Build history of the part. All positions in model axes, mm. Give positions to 0.01 mm unless a question says otherwise; leave off trailing zeros. Order: outer loops, then holes, each group sorted by start corner. A loop starts at its lowest first (then second) coordinate and runs counter-clockwise, first axis right, second up. Notation, with made-up numbers: (51.5, -10) - (98.5, -10) arc R25 cw to (98.5, 13) - close; hole circle Ø5 at (72.25, 52). An arc over 180 degrees is marked (long way). Use a Markdown table: item, result. Add a question column.
(1) Slice it at A-A (y = -449.5). Write the cut outline in (x, z), then the cut area to 3 significant figures.
(2) Slice it at C-C (z = 0.85). Count the separate pieces of the cut face and the enclosed holes in it, then the cut area to 3 significant figures.
(3) Wall check: line 1 (Y direction, x = 454, z = 1.8); line 2 (X direction, y = -454, z = 0.2); line 3 (Y direction, x = 534, z = 1.7). Give the ranges that are in metal, low to high.
(4) Mould opens along Y. For faces 1 (the face through (431, -460, 0)), 2 (the face through (323.605, -459.868, 1.479)) say: +Y half, -Y half, draft (parallel to the pull), parting line (faces both ways), or undercut.
(5) Flat gauge pin, fed straight in: pin 1 (3.5 mm diameter, centred on x = 458.79, y = -436, fed in from -Z). Where does the tip first touch, or does it go through?
(6) Slice it at B-B (x = 480). Write the cut outline in (y, z), then the cut area to 3 significant figures.
from build123d import *

# Parameters (mm, degrees)
SKETCH1_W           = 248
SKETCH1_H           = 78
SKETCH1_R           = 3.05
SKETCH1_W_2         = 24.2
SKETCH1_H_2         = 3.2
SKETCH1_W_3         = 3.2
SKETCH1_H_3         = 20.3
BOSS_EXTRUDE2_DEPTH = 3
SKETCH5_R           = 2.55
CUT_EXTRUDE1_DEPTH  = 10


with BuildPart() as part:
    # Sketch1 → Boss-Extrude2 (new body)
    with BuildSketch(Plane(origin=(0, 0, 0), x_dir=(-1, 0, 0), z_dir=(0, 0, 1))):
        with Locations((-428.787224347, 459)):
            Rectangle(SKETCH1_W, SKETCH1_H)
        with Locations(Location((-338.787224347, 436, 0), (0, 0, 180))):
            Circle(SKETCH1_R, mode=Mode.SUBTRACT)
        with Locations(Location((-368.787224347, 436, 0), (0, 0, 180))):
            Circle(SKETCH1_R, mode=Mode.SUBTRACT)
        with Locations(Location((-428.787224347, 436, 0), (0, 0, 180))):
            Circle(SKETCH1_R, mode=Mode.SUBTRACT)
        with Locations(Location((-398.787224347, 436, 0), (0, 0, 180))):
            Circle(SKETCH1_R, mode=Mode.SUBTRACT)
        with Locations(Location((-488.787224347, 436, 0), (0, 0, 180))):
            Circle(SKETCH1_R, mode=Mode.SUBTRACT)
        with Locations(Location((-458.787224347, 436, 0), (0, 0, 180))):
            Circle(SKETCH1_R, mode=Mode.SUBTRACT)
        with Locations(Location((-458.787224347, 482, 0), (0, 0, 180))):
            Circle(SKETCH1_R, mode=Mode.SUBTRACT)
        with Locations(Location((-428.787224347, 482, 0), (0, 0, 180))):
            Circle(SKETCH1_R, mode=Mode.SUBTRACT)
        with Locations(Location((-398.787224347, 482, 0), (0, 0, 180))):
            Circle(SKETCH1_R, mode=Mode.SUBTRACT)
        with Locations(Location((-368.787224347, 482, 0), (0, 0, 180))):
            Circle(SKETCH1_R, mode=Mode.SUBTRACT)
        with Locations(Location((-338.787224347, 482, 0), (0, 0, 180))):
            Circle(SKETCH1_R, mode=Mode.SUBTRACT)
        with Locations(Location((-320.787224347, 458.7, 0), (0, 0, 180))):
            Circle(SKETCH1_R, mode=Mode.SUBTRACT)
        with Locations(Location((-488.787224347, 482, 0), (0, 0, 180))):
            Circle(SKETCH1_R, mode=Mode.SUBTRACT)
        with Locations(Location((-518.787224347, 436, 0), (0, 0, 180))):
            Circle(SKETCH1_R, mode=Mode.SUBTRACT)
        with Locations(Location((-536.787224347, 459, 0), (0, 0, 180))):
            Circle(SKETCH1_R, mode=Mode.SUBTRACT)
        with Locations(Location((-518.787224347, 482, 0), (0, 0, 180))):
            Circle(SKETCH1_R, mode=Mode.SUBTRACT)
        with Locations((-383.787224347, 491.4)):
            Rectangle(SKETCH1_W_2, SKETCH1_H_2, mode=Mode.SUBTRACT)
        with Locations((-413.787224347, 491.4)):
            Rectangle(SKETCH1_W_2, SKETCH1_H_2, mode=Mode.SUBTRACT)
        with Locations((-353.787224347, 491.4)):
            Rectangle(SKETCH1_W_2, SKETCH1_H_2, mode=Mode.SUBTRACT)
        with Locations((-443.787224347, 491.4)):
            Rectangle(SKETCH1_W_2, SKETCH1_H_2, mode=Mode.SUBTRACT)
        with Locations((-473.787224347, 491.4)):
            Rectangle(SKETCH1_W_2, SKETCH1_H_2, mode=Mode.SUBTRACT)
        with Locations((-503.787224347, 491.4)):
            Rectangle(SKETCH1_W_2, SKETCH1_H_2, mode=Mode.SUBTRACT)
        with Locations((-533.787224347, 491.4)):
            Rectangle(SKETCH1_W_2, SKETCH1_H_2, mode=Mode.SUBTRACT)
        with Locations((-323.787224347, 491.4)):
            Rectangle(SKETCH1_W_2, SKETCH1_H_2, mode=Mode.SUBTRACT)
        with Locations((-313.387224347, 445.55)):
            Rectangle(SKETCH1_W_3, SKETCH1_H_3, mode=Mode.SUBTRACT)
        with Locations((-313.387224347, 471.85)):
            Rectangle(SKETCH1_W_3, SKETCH1_H_3, mode=Mode.SUBTRACT)
        with Locations((-544.187224347, 445.55)):
            Rectangle(SKETCH1_W_3, SKETCH1_H_3, mode=Mode.SUBTRACT)
        with Locations((-544.187224347, 471.85)):
            Rectangle(SKETCH1_W_3, SKETCH1_H_3, mode=Mode.SUBTRACT)
        with Locations((-533.787224347, 426.6)):
            Rectangle(SKETCH1_W_2, SKETCH1_H_2, mode=Mode.SUBTRACT)
        with Locations((-503.787224347, 426.6)):
            Rectangle(SKETCH1_W_2, SKETCH1_H_2, mode=Mode.SUBTRACT)
        with Locations((-473.787224347, 426.6)):
            Rectangle(SKETCH1_W_2, SKETCH1_H_2, mode=Mode.SUBTRACT)
        with Locations((-443.787224347, 426.6)):
            Rectangle(SKETCH1_W_2, SKETCH1_H_2, mode=Mode.SUBTRACT)
        with Locations((-413.787224347, 426.6)):
            Rectangle(SKETCH1_W_2, SKETCH1_H_2, mode=Mode.SUBTRACT)
        with Locations((-383.787224347, 426.6)):
            Rectangle(SKETCH1_W_2, SKETCH1_H_2, mode=Mode.SUBTRACT)
        with Locations((-353.787224347, 426.6)):
            Rectangle(SKETCH1_W_2, SKETCH1_H_2, mode=Mode.SUBTRACT)
        with Locations((-323.787224347, 426.6)):
            Rectangle(SKETCH1_W_2, SKETCH1_H_2, mode=Mode.SUBTRACT)
    extrude(amount=BOSS_EXTRUDE2_DEPTH)

    # Sketch5 → Cut-Extrude1 (cut)
    with BuildSketch(Plane.XY.offset(3)):
        with Locations((353.787224347, -459)):
            Circle(SKETCH5_R)
        with Locations((383.787224347, -459)):
            Circle(SKETCH5_R)
        with Locations((413.787224347, -459)):
            Circle(SKETCH5_R)
        with Locations((443.787224347, -459)):
            Circle(SKETCH5_R)
        with Locations((473.787224347, -459)):
            Circle(SKETCH5_R)
        with Locations((503.787224347, -459)):
            Circle(SKETCH5_R)
    extrude(amount=-CUT_EXTRUDE1_DEPTH, mode=Mode.SUBTRACT)


solid = part.part
Solution:
| question | item | result |
|---|---|---|
| 1 | outline | (304.79, 0) - (311.79, 0) - (311.79, 3) - (304.79, 3) - close; (314.99, 0) - (542.59, 0) - (542.59, 3) - (314.99, 3) - close; (545.79, 0) - (552.79, 0) - (552.79, 3) - (545.79, 3) - close |
| 1 | area | 725 mm2 |
| 2 | separate pieces | 1 |
| 2 | enclosed holes | 42 |
| 2 | area | 17,300 mm2 |
| 3 | line 1 | -498 to -493, -489.8 to -428.2, -425 to -420 |
| 3 | line 2 | 304.79 to 311.79, 314.99 to 542.59, 545.79 to 552.79 |
| 3 | line 3 | -498 to -493, -489.8 to -460.24, -457.76 to -428.2, -425 to -420 |
| 4 | face 1 | draft |
| 4 | face 2 | undercut |
| 5 | pin 1 | through |
| 6 | outline | (-498, 0) - (-493, 0) - (-493, 3) - (-498, 3) - close; (-489.8, 0) - (-428.2, 0) - (-428.2, 3) - (-489.8, 3) - close; (-425, 0) - (-420, 0) - (-420, 3) - (-425, 3) - close |
| 6 | area | 215 mm2 |
